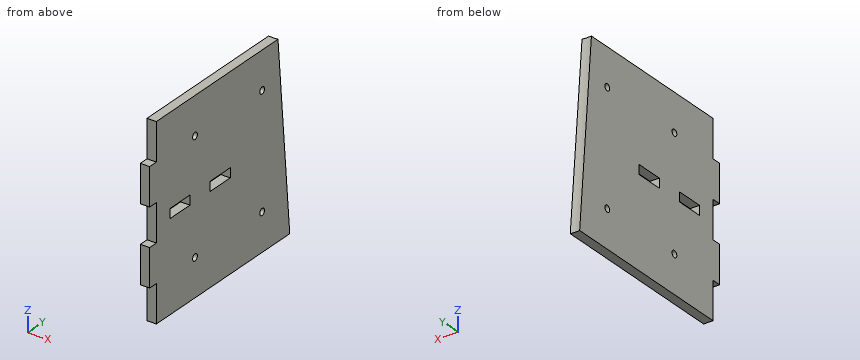
from build123d import *

# Parameters (mm, degrees)
BOSS_EXTRUDE1_OUTLINE_W = 5.08
BOSS_EXTRUDE1_OUTLINE_H = 101.6
BOSS_EXTRUDE1_DEPTH     = 105.948861845
BOSS_EXTRUDE1_START     = 7
BOSS_EXTRUDE1_2_DEPTH   = 104
M3_CLEARANCE_HOLE1_D    = 3.6
SKETCH12_W              = 20.32
SKETCH12_H              = 5.08
CUT_EXTRUDE1_DEPTH      = 147.879296452
SKETCH13_W              = 5.08
SKETCH13_H              = 15.24
CUT_EXTRUDE2_DEPTH      = 147.879296452


with BuildPart() as part:
    # Boss-Extrude1: read off the stored shape, not the designer's step
    # Boss-Extrude1 outline → Boss-Extrude1 (new body)
    with BuildSketch(Plane(origin=(0, 0, 0), x_dir=(1, 0, 0), z_dir=(0, 1, 0))):
        with Locations((2.54, 50.8)):
            Rectangle(BOSS_EXTRUDE1_OUTLINE_W, BOSS_EXTRUDE1_OUTLINE_H)
    extrude(amount=BOSS_EXTRUDE1_DEPTH)

    # Boss-Extrude1 2 outline → Boss-Extrude1 2 (cut)
    with BuildSketch(Plane(origin=(0, 0, 0), x_dir=(1, 0, 0), z_dir=(0, 0.08715574274764448, -0.9961946980917468)).offset(BOSS_EXTRUDE1_START)):
        with BuildLine():
            ThreePointArc((5.08, -96.690670975), (2.54, -96.561403015), (0, -96.690670975))
            Line((0, -96.690670975), (-2, -96.894771203))
            Line((-2, -96.894771203), (-2, -107))
            Line((-2, -107), (7, -107))
            Line((7, -107), (7, -96.886607194))
            Line((7, -96.886607194), (5.08, -96.690670975))
        make_face()
    extrude(amount=BOSS_EXTRUDE1_2_DEPTH, mode=Mode.SUBTRACT)

    # M3 Clearance Hole1 (through all)
    with Locations(Plane(origin=(5.08, 0, 0), x_dir=(0, 0, -1), z_dir=(1, 0, 0))):
        with Locations((81.28, 85.09), (20.32, 85.09), (20.32, 34.29), (81.28, 34.29)):
            Hole(M3_CLEARANCE_HOLE1_D / 2)

    # Sketch12 → Cut-Extrude1 (cut, through all)
    with BuildSketch(Plane(origin=(5.08, 0, 0), x_dir=(0, 0, -1), z_dir=(1, 0, 0))):
        with Locations((91.44, 2.54)):
            Rectangle(SKETCH12_W, SKETCH12_H)
        with Locations((50.8, 2.54)):
            Rectangle(SKETCH12_W, SKETCH12_H)
        with Locations((10.16, 2.54)):
            Rectangle(SKETCH12_W, SKETCH12_H)
    extrude(amount=-CUT_EXTRUDE1_DEPTH, mode=Mode.SUBTRACT)

    # Sketch13 → Cut-Extrude2 (cut, through all)
    with BuildSketch(Plane.ZY):
        with Locations((-50.8, 53.34)):
            Rectangle(SKETCH13_W, SKETCH13_H)
        with Locations((-50.8, 22.86)):
            Rectangle(SKETCH13_W, SKETCH13_H)
    extrude(amount=-CUT_EXTRUDE2_DEPTH, mode=Mode.SUBTRACT)


solid = part.part
Design review of the part built by this model. Coordinates are the model's own, in mm. Round coordinates to 2 decimals unless told otherwise and drop trailing zeros. Order: outer loops, then holes, each group sorted by start corner. A loop starts at its lowest first (then second) coordinate and runs counter-clockwise, first axis right, second up. Notation, with made-up numbers: M -19.75,48 L 13.25,48 A33 cw 13.25,84 Z; hole C -8.75,-5 d11. An arc over 180 degrees is marked long. Answer as CSV lines item,"result". Start each with the question number.
1) Add section B-B (y = 59). Give the boundary of the cut face in (x, z).
2) For pin 1 Ø1.5 at (y, z) = (24.5, -33.5) entering from -X; pin 2 Ø2.5 at (x, z) = (3.5, -89.5) entering from -Y; pin 3 Ø3 at (y, z) = (85.09, -20.32) entering from -X; pin 4 Ø1.5 at (x, y) = (2.5, 2.5) entering from -Z, all flat-tipped, find the tip position at first contact; note any pin that passes through.
3) Wall thickness on line 1 along Z through (x, y) = (1.6, 85.09); line 2 along Z through (x, y) = (1.65, 51); line 3 along Y through (x, z) = (2.3, -56.5): over which ranges is each line inside the solid? List them lowest first. Write a range as [from, to].
4) Add section C-C (x = 2.85). Give the boundary of the cut face in (y, z), then the cut area to 3 significant figures.
5) Add section A-A (y = 85.09). Give the boundary of the cut face in (x, z), then the cut area to 3 significant figures.
Resolved:
1,outline,"M 0,-101.6 L 5.08,-101.6 L 5.08,-53.34 L 0,-53.34 Z; M 0,-48.26 L 5.08,-48.26 L 5.08,0 L 0,0 Z"
2,pin 1,"x = 0"
2,pin 2,"y = 5.08"
2,pin 3,"through"
2,pin 4,"z = -81.28"
3,line 1,"[-101.6, -83.08], [-79.48, -22.12], [-18.52, 0]"
3,line 2,"[-101.6, -53.34], [-48.26, 0]"
3,line 3,"[5.08, 101.87]"
4,outline,"M 0,-81.28 L 5.08,-81.28 L 5.08,-101.6 L 105.82,-101.6 L 96.93,0 L 5.08,0 L 5.08,-20.32 L 0,-20.32 L 0,-40.64 L 5.08,-40.64 L 5.08,-60.96 L 0,-60.96 Z; hole M 15.24,-53.34 L 30.48,-53.34 L 30.48,-48.26 L 15.24,-48.26 Z; hole C 34.29,-81.28 d3.6; hole C 34.29,-20.32 d3.6; hole M 45.72,-53.34 L 60.96,-53.34 L 60.96,-48.26 L 45.72,-48.26 Z; hole C 85.09,-81.28 d3.6; hole C 85.09,-20.32 d3.6"
4,area,"9,790 mm^2"
5,outline,"M 0,-101.6 L 5.08,-101.6 L 5.08,-83.08 L 0,-83.08 Z; M 0,-79.48 L 5.08,-79.48 L 5.08,-22.12 L 0,-22.12 Z; M 0,-18.52 L 5.08,-18.52 L 5.08,0 L 0,0 Z"
5,area,"480 mm^2"
